Verification items for the finished model (mm, model axes). A direction names the side the tool comes from. Coordinates: 2 decimals unless noted, no trailing zeros. Write each loop counter-clockwise with the first axis right and the second up, starting at its lowest first coordinate (ties: lowest second). Pieces come first, ordered by that corner, then holes. Notation, with made-up numbers: M 69,4 L 116,4 A15 ccw 116,28 Z; hole C 16,15 d2. An arc over 180 degrees is marked long. One line per item, written item: value.
```python
from build123d import *

# Parameters (mm, degrees)
SKETCH_1_R               = 3.2
EXTRUDE_1_DEPTH          = 8.5
EXTRUDE_2_DEPTH          = 8.5
PATTERN_CIRCULAR_1_COUNT = 7
PATTERN_CIRCULAR_1_ANGLE = 90
EXTRUDE_3_DEPTH          = 2.5
PATTERN_CIRCULAR_2_COUNT = 19
PATTERN_CIRCULAR_2_ANGLE = 90
CUT_EXTRUDE_1_DEPTH      = 5.5
CUT_EXTRUDE_2_DEPTH      = 5.5


with BuildPart() as part:
    # 스케치1 → 보스-돌출1 (new body)
    with BuildSketch(Plane(origin=(0, 0, 0), x_dir=(1, 0, 0), z_dir=(0, 1, 0))):
        with BuildLine():
            Line((-8.25, -80), (-8.25, -22.5))
            ThreePointArc((-8.25, -22.5), (-5.833630945, -16.666369055), (0, -14.25))
            ThreePointArc((0, -14.25), (10.076271632, -10.076271632), (14.25, 0))
            ThreePointArc((14.25, 0), (16.666369055, 5.833630945), (22.5, 8.25))
            Line((22.5, 8.25), (80, 8.25))
            ThreePointArc((80, 8.25), (85.833630945, 5.833630945), (88.25, 0))
            ThreePointArc((88.25, 0), (62.40217344, -62.40217344), (0, -88.25))
            ThreePointArc((0, -88.25), (-5.833630945, -85.833630945), (-8.25, -80))
        make_face()
        with Locations((58.75, -33.75)):
            Circle(SKETCH_1_R, mode=Mode.SUBTRACT)
        with Locations((33.75, -58.75)):
            Circle(SKETCH_1_R, mode=Mode.SUBTRACT)
        with Locations((8.75, -33.75)):
            Circle(SKETCH_1_R, mode=Mode.SUBTRACT)
        with Locations((33.75, -8.75)):
            Circle(SKETCH_1_R, mode=Mode.SUBTRACT)
        with BuildLine():
            ThreePointArc((0, -19.25), (-3.25, -22.5), (0, -25.75))
            ThreePointArc((0, -25.75), (18.207999616, -18.207999616), (25.75, 0))
            ThreePointArc((25.75, 0), (22.5, 3.25), (19.25, 0))
            ThreePointArc((19.25, 0), (13.611805538, -13.611805538), (0, -19.25))
        make_face(mode=Mode.SUBTRACT)
        with BuildLine():
            ThreePointArc((0, -76.75), (-3.25, -80), (0, -83.25))
            ThreePointArc((0, -83.25), (58.866639534, -58.866639534), (83.25, 0))
            ThreePointArc((83.25, 0), (80, 3.25), (76.75, 0))
            ThreePointArc((76.75, 0), (54.270445456, -54.270445456), (0, -76.75))
        make_face(mode=Mode.SUBTRACT)
    extrude(amount=EXTRUDE_1_DEPTH)

    # 스케치2 → 보스-돌출2 (add)
    with BuildSketch(Plane(origin=(0, 8.5, 0), x_dir=(1, 0, 0), z_dir=(0, 1, 0))):
        with BuildLine():
            Line((0.458146835, -87.498800572), (0.463382799, -88.498786864))
            ThreePointArc((0.463382799, -88.498786864), (0, -88.5), (-0.463382799, -88.498786864))
            Line((-0.463382799, -88.498786864), (-0.458146835, -87.498800572))
            ThreePointArc((-0.458146835, -87.498800572), (0, -87.5), (0.458146835, -87.498800572))
        make_face()
    extrude_2 = extrude(amount=-EXTRUDE_2_DEPTH)

    # 원형 패턴1: 보스-돌출2 ×7 about axis
    pattern_circular_1_axis = Axis((0, 0, 0), (0, 1, 0))
    for i in range(1, PATTERN_CIRCULAR_1_COUNT):
        add(extrude_2.rotate(pattern_circular_1_axis, i * PATTERN_CIRCULAR_1_ANGLE / (PATTERN_CIRCULAR_1_COUNT - 1)))

    # 스케치6 → 보스-돌출3 (add)
    with BuildSketch(Plane.XZ):
        with BuildLine():
            Line((88.498786864, 0.463382799), (87.998793718, 0.460764817))
            ThreePointArc((87.998793718, 0.460764817), (88, 0), (87.998793718, -0.460764817))
            Line((87.998793718, -0.460764817), (88.498786864, -0.463382799))
            ThreePointArc((88.498786864, -0.463382799), (88.5, 0), (88.498786864, 0.463382799))
        make_face()
    extrude_3 = extrude(amount=-EXTRUDE_3_DEPTH)

    # 원형 패턴2: 보스-돌출3 ×19 about axis
    pattern_circular_2_axis = Axis((0, 8.5, 0), (0, -1, 0))
    for i in range(1, PATTERN_CIRCULAR_2_COUNT):
        add(extrude_3.rotate(pattern_circular_2_axis, i * PATTERN_CIRCULAR_2_ANGLE / (PATTERN_CIRCULAR_2_COUNT - 1)))

    # 스케치7 → 컷-돌출1 (cut)
    with BuildSketch(Plane.XZ):
        Polygon((26.650803984, 56.831298374), (35.668701626, 51.650803984), (40.849196016, 60.668701626), (31.831298374, 65.849196016), align=None)
        Polygon((51.650803984, 35.668701626), (56.831298374, 26.650803984), (65.849196016, 31.831298374), (60.668701626, 40.849196016), align=None)
        Polygon((30.021419355, 2.411412904), (40.088587096, 5.021419355), (37.478580645, 15.088587096), (27.411412904, 12.478580645), align=None)
        Polygon((2.411412904, 30.021419355), (12.478580645, 27.411412904), (15.088587096, 37.478580645), (5.021419355, 40.088587096), align=None)
    extrude(amount=-CUT_EXTRUDE_1_DEPTH, mode=Mode.SUBTRACT)

    # 스케치8 → 컷-돌출2 (cut)
    with BuildSketch(Plane(origin=(0, 8.5, 0), x_dir=(1, 0, 0), z_dir=(0, 1, 0))):
        with BuildLine():
            ThreePointArc((27.75, 0), (22.5, 5.25), (17.25, 0))
            ThreePointArc((17.25, 0), (12.197591975, -12.197591975), (0, -17.25))
            ThreePointArc((0, -17.25), (-5.25, -22.5), (0, -27.75))
            ThreePointArc((0, -27.75), (19.622213178, -19.622213178), (27.75, 0))
        make_face()
        with BuildLine():
            ThreePointArc((85.25, 0), (80, 5.25), (74.75, 0))
            ThreePointArc((74.75, 0), (52.856231894, -52.856231894), (0, -74.75))
            ThreePointArc((0, -74.75), (-5.25, -80), (0, -85.25))
            ThreePointArc((0, -85.25), (60.280853096, -60.280853096), (85.25, 0))
        make_face()
    extrude(amount=-CUT_EXTRUDE_2_DEPTH, mode=Mode.SUBTRACT)


solid = part.part
```
Item 1: Access from +Z, -Z, +X, -X, +Y, -Y to the whole of each face (thin tool, end or side, straight path). Record for faces 1 (the face through (-8.25, 4, 52)), 2 (the face through (32.515, 2.712, 13.802)), 3 (the face through (80.12, 5.79, -5.25)), 4 (the face through (13.76, 1.48, 13.46)).
The answers:
face 1: +Z, -Z, -X, +Y, -Y
face 2: -Y
face 3: +Y
face 4: +Y, -Y
Item 2: Scan lines: line 1 (X direction, y = 6.6, z = 33.75); line 2 (X direction, y = 6.2, z = 8.75); line 3 (Z direction, x = 4.5, y = 5.75). Record each from-to range of solid material in increasing order.
The answers:
line 1: x = -8.25 to 5.55, 11.95 to 55.55, 61.95 to 66.7, 78.28 to 81.54
line 2: x = 11.25 to 14.87, 26.33 to 30.55, 36.95 to 74.24, 84.8 to 87.82
line 3: z = 13.52 to 16.65, 27.38 to 74.61, 85.13 to 88.14
Item 3: Cross-section at B-B, the plane z = 58.75. Enter the section's corners in (x, y).
The answers:
outline: M -8.25,0 L 27.75,0 L 27.75,5.5 L 30.55,5.5 L 30.55,8.5 L -8.25,8.5 Z; M 36.95,5.5 L 39.75,5.5 L 39.75,0 L 49.39,0 L 49.39,3 L 46.22,3 L 46.22,8.5 L 36.95,8.5 Z; M 58.98,0 L 65.85,0 L 65.85,8.5 L 61.77,8.5 L 61.77,3 L 58.98,3 Z
Item 4: Cross-section at C-C, the plane x = 58.75. Enter the section's corners in (y, z).
The answers:
outline: M 0,-8.25 L 8.5,-8.25 L 8.5,30.55 L 5.5,30.55 L 5.5,27.75 L 0,27.75 Z; M 0,39.75 L 5.5,39.75 L 5.5,36.95 L 8.5,36.95 L 8.5,46.22 L 3,46.22 L 3,49.39 L 0,49.39 Z; M 0,58.98 L 3,58.98 L 3,61.77 L 8.5,61.77 L 8.5,65.85 L 0,65.85 Z
Item 5: Draft check along X on faces 5 (the face through (85.604, 4.19, -6.055)), 6 (the face through (-3.25, 1.48, 79.93)), 7 (the face through (9.96, 4.19, 10.19)), 8 (the face through (56.223, 2.712, 38.295)). Enter one of: released by +X, released by -X, zero draft, split by the parting line, or undercut.
The answers:
face 5: released by +X
face 6: undercut
face 7: released by -X
face 8: undercut
Item 6: Cross-section at A-A, the plane x = 33.75. Enter the section's corners in (y, z).
The answers:
outline: M 0,-8.25 L 8.5,-8.25 L 8.5,5.55 L 5.5,5.55 L 5.5,3.38 L 0,3.38 Z; M 0,14.12 L 5.5,14.12 L 5.5,11.95 L 8.5,11.95 L 8.5,55.55 L 5.5,55.55 L 5.5,52.75 L 0,52.75 Z; M 0,64.75 L 5.5,64.75 L 5.5,61.95 L 8.5,61.95 L 8.5,66.7 L 3,66.7 L 3,68.93 L 0,68.93 Z; M 0,76.1 L 3,76.1 L 3,78.28 L 8.5,78.28 L 8.5,81.54 L 0,81.54 Z
Item 7: Go/stop test with flat-tipped pins: P1, Ø5, axis at x = 64, y = 3, coming from the +Z side; P2, Ø0.6, axis at x = 56.5, z = 68, coming from the +Y side; P3, Ø1.5, axis at x = 55, y = 3.5, coming from the +Z side; P4, Ø8.5, axis at x = 58.75, z = 33.75, coming from the -Y side. Record where each tip stops, or that it passes through.
The answers:
P1: stops at z = 63.29
P2: stops at y = 8.5
P3: stops at z = 69.61
P4: stops at y = 5.5
